Input: dimensioned drawing with shaded views. Units: mm. Origin: part minimum x, y, z. A direction names the side the tool comes from. Give positions to 0.01 mm unless a question says otherwise; leave off trailing zeros. Write each loop counter-clockwise with the first axis right and the second up, starting at its lowest first coordinate (ties: lowest second). Pieces come first, ordered by that corner, then holes.
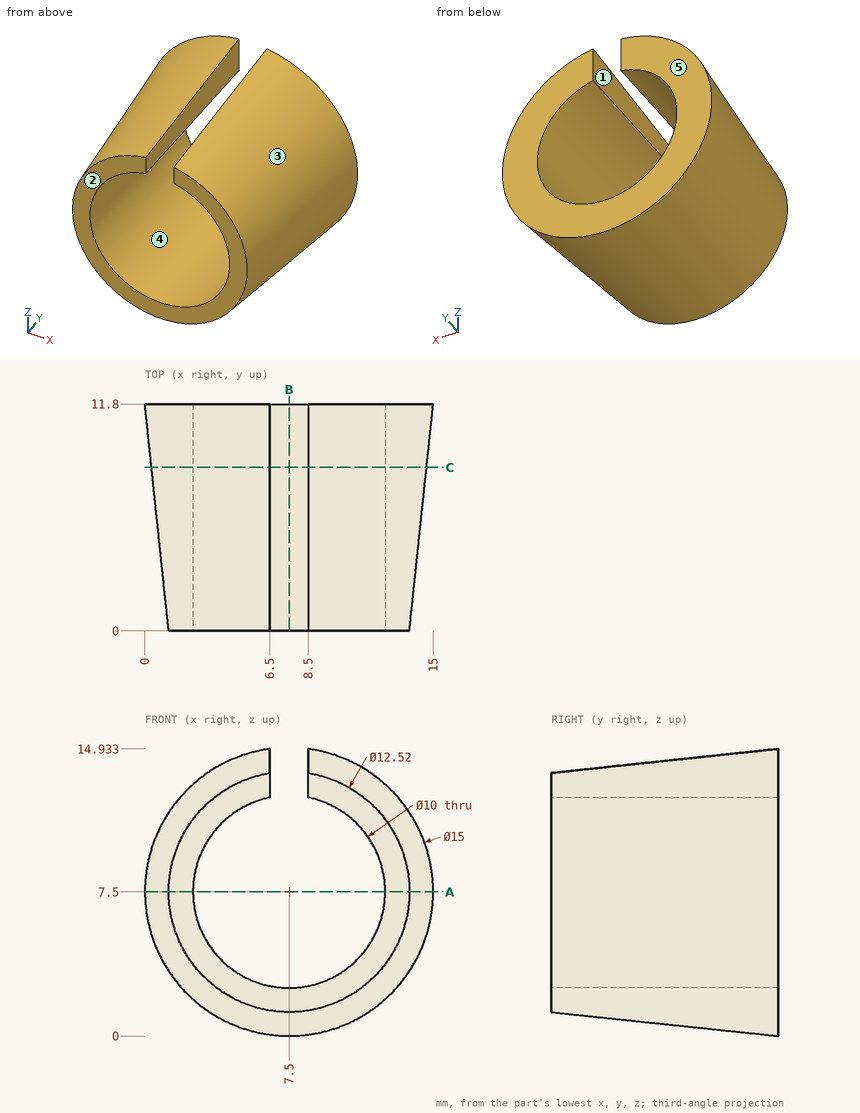
Item 1: Section A-A, the plane z = 7.5. Return the cut outline in (x, y).
Found:
outline: (0, 11.8) - (1.24, 0) - (2.5, 0) - (2.5, 11.8) - close; (12.5, 0) - (13.76, 0) - (15, 11.8) - (12.5, 11.8) - close
Item 2: Section B-B, the plane x = 7.5. Return the cut outline in (y, z), plus the area to 3 significant figures.
Found:
outline: (0, 1.24) - (11.8, 0) - (11.8, 2.5) - (0, 2.5) - close
area: 22.2 mm2
Item 3: Section C-C, the plane y = 8.5. Return the cut outline in (x, z).
Found:
outline: (6.5, 12.4) - (6.5, 14.58) arc R7.15 ccw (long way) to (8.5, 14.58) - (8.5, 12.4) arc R5 cw (long way) to start
Item 4: Pull-direction query (X, two-part tool) for the marked faces 3, 4 and 5; classes: +X half, -X half, draft (parallel to the pull), parting line (faces both ways), or undercut.
Found:
face 3: parting line
face 4: undercut
face 5: draft
Item 5: Reachability of the marked faces 1 and 2 from +Z, -Z, +X, -X, +Y, -Y: full face, straight path, thin tool, end or side. Return the list, or none.
Found:
face 1: +Z, +Y, -Y
face 2: +Z, -Z, +X, -X, -Y
Item 6: Pin query (flat end, axial travel): pin 1 Ø1 at (y, z) = (10, 12.5) entering from -X; pin 2 Ø5 at (x, z) = (11, 10) entering from -Y; pin 3 Ø6 at (y, z) = (5.5, 6) entering from +X; pin 4 Ø6 at (x, y) = (11.5, 2) entering from +Z. Return the tip coordinate at first contact, or that it passes through.
Found:
pin 1: stops at x = 1.73
pin 2: stops at y = 0
pin 3: stops at x = 14.62
pin 4: stops at z = 13.98
Item 7: Line query: L1, parallel to X at y = 2.5, z = 7.25; L2, parallel to X at y = 10, z = 9.25 (1 decimal); L3, parallel to Z at x = 9.25, y = 5.5 (1 decimal). Output: solid intervals per line, ascending.
Found:
L1: x = 0.98 to 2.51, 12.49 to 14.02
L2: x = 0.4 to 2.8, 12.2 to 14.6
L3: z = 0.9 to 2.8, 12.2 to 14.1
